For this review, take the finished solid that the model builds, in its own axes (mm). A direction names the side the tool comes from. Coordinates: 2 decimals unless noted, no trailing zeros. Loops run counter-clockwise (first coordinate to the right, second up) from the corner with the lowest first, then second, coordinate; pieces in that order, holes last.
```python
from build123d import *

# Parameters (mm, degrees)
AUFSATZ_LINEAR_AUSTRAGEN1_DEPTH      = 35
AUFSATZ_LINEAR_AUSTRAGEN1_DEPTH_BACK = 35
SKIZZE1_R                            = 20
SKIZZE2_W                            = 50
SKIZZE2_H                            = 35
AUFSATZ_LINEAR_AUSTRAGEN2_DEPTH      = 550
AUFSATZ_LINEAR_AUSTRAGEN3_DEPTH      = 10
SCHNITT_LINEAR_AUSTRAGEN1_REACH      = 598.956
SKIZZE4_R                            = 6
SKIZZE5_R                            = 14
AUFSATZ_LINEAR_AUSTRAGEN4_DEPTH      = 40
VERRUNDUNG1_R                        = 9
FASE2_SIZE                           = 20


with BuildPart() as part:
    # Skizze1 → Aufsatz-Linear austragen1 (new, two sides: drawn at the far end of the back side and taken through both)
    with BuildSketch(Plane(origin=(0, 0, 0), x_dir=(0, 0, -1), z_dir=(1, 0, 0)).offset(-AUFSATZ_LINEAR_AUSTRAGEN1_DEPTH_BACK)):
        Circle(SKIZZE1_R)
    extrude(amount=AUFSATZ_LINEAR_AUSTRAGEN1_DEPTH + AUFSATZ_LINEAR_AUSTRAGEN1_DEPTH_BACK)

    # Skizze2 → Aufsatz-Linear austragen2 (add)
    with BuildSketch(Plane.XY):
        Rectangle(SKIZZE2_W, SKIZZE2_H)
    extrude(amount=AUFSATZ_LINEAR_AUSTRAGEN2_DEPTH)

    # Skizze3 → Aufsatz-Linear austragen3 (add)
    with BuildSketch(Plane.ZY.offset(25)):
        with BuildLine():
            Line((550, 17.5), (525, 17.5))
            ThreePointArc((525, 17.5), (507.5, 0), (525, -17.5))
            Line((525, -17.5), (550, -17.5))
            Line((550, -17.5), (575, -17.5))
            ThreePointArc((575, -17.5), (592.5, 0), (575, 17.5))
            Line((575, 17.5), (550, 17.5))
        make_face()
    aufsatz_linear_austragen3 = extrude(amount=AUFSATZ_LINEAR_AUSTRAGEN3_DEPTH)

    # Skizze4 → Schnitt-Linear austragen1 (cut, up to next)
    with BuildSketch(Plane.ZY.offset(35), mode=Mode.PRIVATE) as schnitt_linear_austragen1_sk1:
        with Locations(Location((575, 0, 0), (0, 0, 270))):
            Circle(SKIZZE4_R)
    schnitt_linear_austragen1_tool1 = extrude(schnitt_linear_austragen1_sk1.sketch, amount=-SCHNITT_LINEAR_AUSTRAGEN1_REACH, mode=Mode.PRIVATE) & part.part
    schnitt_linear_austragen1 = schnitt_linear_austragen1_tool1.solids().sort_by_distance((-35, 0, 575))[0]
    add(schnitt_linear_austragen1, mode=Mode.SUBTRACT)

    # Spiegeln1: Aufsatz-Linear austragen3, Schnitt-Linear austragen1 across plane
    add(aufsatz_linear_austragen3.mirror(Plane(origin=(0, 0, 0), x_dir=(0, 0, 1), z_dir=(1, 0, 0))))
    add(schnitt_linear_austragen1.mirror(Plane(origin=(0, 0, 0), x_dir=(0, 0, 1), z_dir=(1, 0, 0))), mode=Mode.SUBTRACT)

    # Skizze5 → Aufsatz-Linear austragen4 (add)
    with BuildSketch(Plane(origin=(35, 0, 0), x_dir=(0, 0, -1), z_dir=(1, 0, 0))):
        with Locations(Location((-575, 0, 0), (0, 0, 90))):
            Circle(SKIZZE5_R)
    extrude(amount=AUFSATZ_LINEAR_AUSTRAGEN4_DEPTH)

    # Verrundung1
    verrundung1_edges = [part.edges().sort_by_distance(p)[0] for p in [
        (-25, 17.5, 267.341229183),
        (-25, -17.5, 267.341229183),
        (25, 17.5, 267.341229183),
        (25, -17.5, 267.341229183),
    ]]
    fillet(verrundung1_edges, radius=VERRUNDUNG1_R)

    # Fase2
    # the kernel refuses this chamfer: 20 mm, written as the material it takes off along each edge
    with BuildSketch(Plane(origin=(25, -17.5, 550), x_dir=(0, -0.027495876610586282, -0.9996219169112968), z_dir=(-1, 0, 0))) as fase2_piece_1:
        Polygon((FASE2_SIZE * 0.999621916911, -FASE2_SIZE * 0.0274958766106), (-FASE2_SIZE * 0.0274958766106, -FASE2_SIZE * 0.999621916911), (0, 0), align=None)
    extrude(amount=50, mode=Mode.SUBTRACT)
    with BuildSketch(Plane(origin=(-25, 17.5, 550), x_dir=(0, -0.9996219169112968, 0.0274958766105877), z_dir=(1, 0, 0))) as fase2_piece_2:
        Polygon((FASE2_SIZE * 0.999621916911, FASE2_SIZE * 0.0274958766106), (-FASE2_SIZE * 0.0274958766106, FASE2_SIZE * 0.999621916911), (0, 0), align=None)
    extrude(amount=50, mode=Mode.SUBTRACT)


solid = part.part
```
Q1. Wall thickness on probe 1 along Z at (x, y) = (29.25, 0); probe 2 along Y at (x, z) = (-29.25, 575); probe 3 along X at (y, z) = (-12, 541): over which ranges is each line inside the solid? List them lowest first.
Q2. Consider section B-B (x = 53). State the section outline as (y, z) points.
Q3. The part is to be moulded in two halves that separate along Z. For faces 1 (the face through (35, 0, 575)), 2 (the face through (-29.93, -0.385, 592.496)), 3 (the face through (-30.07, 0.78, 580.95)), 4 (the face through (0, 17.5, 296)), say which applies: +Z half, -Z half, draft (parallel to the pull), parting line (faces both ways), or undercut.
Q4. Consider section A-A (z = 458). State the section outline as (x, y) points, then the cut area to 3 significant figures.
Q5. Machinability: for faces 5 (the face through (35, 0, 0)), 6 (the face through (-0.4, 8.6, 538.9)), 7 (the face through (30.07, 0.78, 580.95)), 8 (the face through (0, -17.5, 288)), which of the approach directions +Z, -Z, +X, -X, +Y, -Y give a long, thin tool a straight path to every point of the face, cutting with its end or side? Answer none if there is none.
Q6. Consider section C-C (z = 0). State the section outline as (x, y) points.
Q7. For pin 1 Ø17.5 at (y, z) = (7, 552) entering from +X; pin 2 Ø5 at (y, z) = (-13.5, 455) entering from +X; pin 3 Ø12 at (x, z) = (25.5, 372) entering from +Y; pin 4 Ø19 at (y, z) = (0, 575) entering from -X, all flat-tipped, find the tip position at first contact; note any pin that passes through.
Model answer:
1. probe 1: z = -20 to 20, 507.5 to 569, 581 to 592.5
1. probe 2: y = -17.5 to -6, 6 to 17.5
1. probe 3: x = -35 to -25, 25 to 35
2. outline: circle Ø28 at (0, 575)
3. face 1: undercut
3. face 2: +Z half
3. face 3: undercut
3. face 4: draft
4. outline: (-25, -8.5) arc R9 ccw to (-16, -17.5) - (16, -17.5) arc R9 ccw to (25, -8.5) - (25, 8.5) arc R9 ccw to (16, 17.5) - (-16, 17.5) arc R9 ccw to (-25, 8.5) - close
4. area: 1,680 mm2
5. face 5: -Z, +X, +Y, -Y
5. face 6: +Z, +Y
5. face 7: -X
5. face 8: +Z, +X, -X, -Y
6. outline: (-35, -20) - (35, -20) - (35, 20) - (-35, 20) - close
7. pin 1: stops at x = 35
7. pin 2: stops at x = 24.65
7. pin 3: stops at y = 16.79
7. pin 4: stops at x = -35
